Design review of the part built by this model. Coordinates are the model's own, in mm. A direction names the side the tool comes from. Give positions to 0.01 mm unless a question says otherwise; leave off trailing zeros. Loops run counter-clockwise (first coordinate to the right, second up) from the corner with the lowest first, then second, coordinate; pieces in that order, holes last. Notation, with made-up numbers: (-5.75, -13.5) - (30.25, -13.5) arc R15 ccw to (30.25, 6.5) - close; hole circle Ø6 at (-3, 58.25). An arc over 180 degrees is marked (long way). Write each question's results on one line, items separated by ' | '.
```python
from build123d import *

# Parameters (mm, degrees)
BOSS_EXTRUDE1_START = 15
BOSS_EXTRUDE1_DEPTH = 75
SKETCH2_W           = 107
SKETCH2_H           = 29
CUT_EXTRUDE1_DEPTH  = 123.079123932
CUT_EXTRUDE12_START = -29.5
CUT_EXTRUDE12_DEPTH = 29.5
SKETCH16_R          = 1.875
CUT_EXTRUDE13_DEPTH = 5
SKETCH17_W          = 46
SKETCH17_H          = 117
CUT_EXTRUDE14_DEPTH = 11.15
SKETCH14_R          = 1.93
CUT_EXTRUDE10_DEPTH = 6.5
FILLET1_R           = 3
BOSS_EXTRUDE3_DEPTH = 5
SKETCH21_R          = 1.375
CUT_EXTRUDE15_DEPTH = 50.5
SKETCH22_R          = 2.5
CUT_EXTRUDE16_DEPTH = 32.85
SKETCH23_R          = 1.93
CUT_EXTRUDE17_DEPTH = 4


with BuildPart() as part:
    # Sketch1 → Boss-Extrude1 (new body)
    with BuildSketch(Plane(origin=(0, 0, 0), x_dir=(0, 0, -1), z_dir=(1, 0, 0)).offset(BOSS_EXTRUDE1_START)):
        with BuildLine():
            Line((-68.626974957, 15.5), (-58.5, 15.5))
            Line((-58.5, 15.5), (-58.5, 27.48087198))
            ThreePointArc((-58.5, 27.48087198), (-66.444952459, 31.270691326), (-75.182099647, 32.341793222))
            ThreePointArc((-75.182099647, 32.341793222), (-75.739500667, 40.338834406), (-75.44865804, 48.35))
            Line((-75.44865804, 48.35), (-58.5, 48.35))
            Line((-58.5, 48.35), (-58.5, 59.5))
            Line((-58.5, 59.5), (58.5, 59.5))
            Line((58.5, 59.5), (58.5, 48.35))
            Line((58.5, 48.35), (75.44865804, 48.35))
            ThreePointArc((75.44865804, 48.35), (75.739500667, 40.338834406), (75.182099647, 32.341793222))
            ThreePointArc((75.182099647, 32.341793222), (66.444952459, 31.270691326), (58.5, 27.48087198))
            Line((58.5, 27.48087198), (58.5, 15.5))
            Line((58.5, 15.5), (68.626974957, 15.5))
            Line((68.626974957, 15.5), (68.626974957, 10.5))
            Line((68.626974957, 10.5), (-68.626974957, 10.5))
            Line((-68.626974957, 10.5), (-68.626974957, 15.5))
        make_face()
    extrude(amount=BOSS_EXTRUDE1_DEPTH)

    # Sketch2 → Cut-Extrude1 (cut, through all)
    with BuildSketch(Plane(origin=(90, 0, 0), x_dir=(0, 0, -1), z_dir=(1, 0, 0))):
        with Locations((0, 25)):
            Rectangle(SKETCH2_W, SKETCH2_H)
    extrude(amount=-CUT_EXTRUDE1_DEPTH, mode=Mode.SUBTRACT)

    # Sketch9 → Cut-Extrude12 (cut)
    with BuildSketch(Plane(origin=(90, 0, 0), x_dir=(0, 0, -1), z_dir=(1, 0, 0)).offset(CUT_EXTRUDE12_START)):
        with BuildLine():
            Line((-58.5, 27.48087198), (-58.5, 48.35))
            Line((-58.5, 48.35), (-75.44865804, 48.35))
            ThreePointArc((-75.44865804, 48.35), (-75.739500667, 40.338834406), (-75.182099647, 32.341793222))
            ThreePointArc((-75.182099647, 32.341793222), (-66.444952459, 31.270691326), (-58.5, 27.48087198))
        make_face()
        with BuildLine():
            Line((58.5, 27.48087198), (58.5, 48.35))
            Line((58.5, 48.35), (75.44865804, 48.35))
            ThreePointArc((75.44865804, 48.35), (75.739500667, 40.338834406), (75.182099647, 32.341793222))
            ThreePointArc((75.182099647, 32.341793222), (66.444952459, 31.270691326), (58.5, 27.48087198))
        make_face()
    extrude(amount=CUT_EXTRUDE12_DEPTH, mode=Mode.SUBTRACT)

    # Sketch16 → Cut-Extrude13 (cut)
    with BuildSketch(Plane.XZ.offset(-10.5)):
        with Locations(Location((27.45, -62.5, 0), (0, 0, 270))):
            Circle(SKETCH16_R)
        with Locations(Location((72.45, -62.5, 0), (0, 0, 270))):
            Circle(SKETCH16_R)
    cut_extrude13 = extrude(amount=-CUT_EXTRUDE13_DEPTH, mode=Mode.SUBTRACT)

    # Mirror2: Cut-Extrude13 across plane
    add(cut_extrude13.mirror(Plane.XY), mode=Mode.SUBTRACT)

    # Sketch17 → Cut-Extrude14 (cut)
    with BuildSketch(Plane(origin=(0, 59.5, 0), x_dir=(1, 0, 0), z_dir=(0, 1, 0))):
        with Locations((23, 0)):
            Rectangle(SKETCH17_W, SKETCH17_H)
    extrude(amount=-CUT_EXTRUDE14_DEPTH, mode=Mode.SUBTRACT)

    # Sketch14 → Cut-Extrude10 (cut)
    with BuildSketch(Plane(origin=(0, 59.5, 0), x_dir=(1, 0, 0), z_dir=(0, 1, 0))):
        with Locations(Location((49.1, 38.1, 0), (0, 0, 270))):
            Circle(SKETCH14_R)
        with Locations(Location((49.1, -38.1, 0), (0, 0, 270))):
            Circle(SKETCH14_R)
    extrude(amount=-CUT_EXTRUDE10_DEPTH, mode=Mode.SUBTRACT)

    # Fillet1
    fillet1_edges = [part.edges().sort_by_distance(p)[0] for p in [
        (90, 13, 68.626974957),
        (15, 13, -68.626974957),
        (15, 13, 68.626974957),
        (68, 59.5, 58.5),
        (68, 59.5, -58.5),
        (90, 13, -68.626974957),
        (37.75, 32.341793222, 75.182099647),
        (37.75, 48.35, 75.44865804),
        (37.75, 32.341793222, -75.182099647),
        (37.75, 27.48087198, -58.5),
        (37.75, 27.48087198, 58.5),
    ]]
    fillet(fillet1_edges, radius=FILLET1_R)

    # Sketch20 → Boss-Extrude3 (add)
    with BuildSketch(Plane(origin=(60.5, 0, 0), x_dir=(0, 0, -1), z_dir=(1, 0, 0))):
        with BuildLine():
            Line((75.44865804, 48.35), (58.5, 48.35))
            Line((58.5, 48.35), (58.5, 25.852098922))
            ThreePointArc((58.5, 25.852098922), (58.887094237, 27.326115025), (59.948482315, 28.41974237))
            ThreePointArc((59.948482315, 28.41974237), (66.053139575, 31.15333873), (72.638618282, 32.324175832))
            ThreePointArc((72.638618282, 32.324175832), (74.564449947, 33.163853344), (75.467231088, 35.060922699))
            ThreePointArc((75.467231088, 35.060922699), (75.749926018, 41.705869428), (75.44865804, 48.35))
        make_face()
    boss_extrude3 = extrude(amount=BOSS_EXTRUDE3_DEPTH)

    # Mirror4: Boss-Extrude3 across plane
    add(boss_extrude3.mirror(Plane.XY))

    # Sketch21 → Cut-Extrude15 (cut)
    with BuildSketch(Plane(origin=(65.5, 0, 0), x_dir=(0, 0, -1), z_dir=(1, 0, 0))):
        with Locations((75.749926018, 41.705869428)):
            Circle(SKETCH21_R)
    extrude(amount=-CUT_EXTRUDE15_DEPTH, mode=Mode.SUBTRACT)

    # Sketch22 → Cut-Extrude16 (cut)
    with BuildSketch(Plane(origin=(0, 15.5, 0), x_dir=(1, 0, 0), z_dir=(0, 1, 0))):
        with Locations(Location((27.45, -62.5, 0), (0, 0, 90))):
            Circle(SKETCH22_R)
    cut_extrude16 = extrude(amount=CUT_EXTRUDE16_DEPTH, mode=Mode.SUBTRACT)

    # Mirror5: Cut-Extrude16 across plane
    add(cut_extrude16.mirror(Plane.XY), mode=Mode.SUBTRACT)

    # Sketch23 → Cut-Extrude17 (cut)
    with BuildSketch(Plane(origin=(46, 2.35, 0), x_dir=(0, 1, 0), z_dir=(-1, 0, 0))):
        with Locations(Location((55.15, 54.5, 0), (0, 0, 270))):
            Circle(SKETCH23_R)
        with Locations(Location((55.15, -54.5, 0), (0, 0, 270))):
            Circle(SKETCH23_R)
    extrude(amount=-CUT_EXTRUDE17_DEPTH, mode=Mode.SUBTRACT)


solid = part.part
```
Item 1: Wall thickness on probe 1 along X at (y, z) = (14.05, 62.5) (3 decimals); probe 2 along X at (y, z) = (44.25, 62.5); probe 3 along Z at (x, y) = (85, 32): over which ranges is each line inside the solid? List them lowest first.
Output values:
probe 1: x = 15 to 25.575, 29.325 to 70.575, 74.325 to 90 | probe 2: x = 15 to 24.95, 29.95 to 65.5 | probe 3: z = -58.5 to -53.5, 53.5 to 58.5
Item 2: We need section A-A on x = 72.45. Give the boundary of the cut face in (y, z) (3 decimals), then the cut area to 3 significant figures.
Output values:
outline: (10.5, -68.627) - (15.5, -68.627) - (15.5, -64.375) - (10.5, -64.375) - close; (10.5, -60.625) - (15.5, -60.625) - (15.5, -58.5) - (56.5, -58.5) arc R3 ccw to (59.5, -55.5) - (59.5, 55.5) arc R3 ccw to (56.5, 58.5) - (15.5, 58.5) - (15.5, 60.625) - (10.5, 60.625) - (10.5, 53.5) - (39.5, 53.5) - (39.5, -53.5) - (10.5, -53.5) - close; (10.5, 64.375) - (15.5, 64.375) - (15.5, 68.627) - (10.5, 68.627) - close | area: 2,690 mm²
Item 3: Draft analysis for pull direction X (two halves, no side actions). For faces 1 (the face through (52, 13, -68.627)), 2 (the face through (26.73, 12.96, 64.23)), 3 (the face through (50, 58, -55)), 4 (the face through (65.5, 40, 67)), state which applies: +X half, -X half, draft (parallel to the pull), parting line (faces both ways), or undercut.
Output values:
face 1: draft | face 2: undercut | face 3: -X half | face 4: +X half
Item 4: We need section B-B on y = 21. Give the boundary of the cut face in (x, z).
Output values:
outline: (15, -58.5) - (90, -58.5) - (90, -53.5) - (15, -53.5) - close; (15, 53.5) - (90, 53.5) - (90, 58.5) - (15, 58.5) - close
Item 5: We need section C-C on z = -6. Give the boundary of the cut face in (x, y).
Output values:
outline: (15, 39.5) - (90, 39.5) - (90, 59.5) - (46, 59.5) - (46, 48.35) - (15, 48.35) - close
Item 6: Clearance check with flat-ended pins moving along their axes: P1, Ø12.5, axis at x = 67.5, y = 33.5, coming from the +Z side; P2, Ø1.5, axis at x = 43.5, y = 12.5, coming from the +Z side; P3, Ø12.5, axis at x = 36, y = 28, coming from the -Z side; P4, Ø3, axis at x = 27.45, z = -62.5, coming from the -Y side. State where each tip first meets the part, or that it passes through.
Output values:
P1: stops at z = 75.72 | P2: stops at z = 68.63 | P3: stops at z = -75.28 | P4: passes through
Item 7: We need section D-D on z = -62.5. Give the boundary of the cut face in (x, y) (3 decimals), then the cut area to 3 significant figures.
Output values:
outline: (15, 10.5) - (25.575, 10.5) - (25.575, 15.5) - (15, 15.5) - close; (15, 29.783) - (24.95, 29.783) - (24.95, 48.35) - (15, 48.35) - close; (29.325, 10.5) - (70.575, 10.5) - (70.575, 15.5) - (29.325, 15.5) - close; (29.95, 29.783) - (65.5, 29.783) - (65.5, 48.35) - (29.95, 48.35) - close; (74.325, 10.5) - (90, 10.5) - (90, 15.5) - (74.325, 15.5) - close | area: 1,180 mm²
Item 8: Tool access review of faces 5 (the face through (50.404, 56.296, 36.678)), 6 (the face through (60.5, 48, 75)), 7 (the face through (52, 15.5, 64)), 8 (the face through (53, 25, 53.5)), 9 (the face through (15.9, 13.04, 67.77)): name each direction out of +Z, -Z, +X, -X, +Y, -Y from which nothing blocks a thin tool from reaching the whole face with its end or side.
Output values:
face 5: +Y | face 6: +Z, -X, +Y | face 7: +Z, +X, -X | face 8: +X, -X, -Y | face 9: +Z, -X, -Y
